Autodesk Inventor part; units mm, degrees
ref_plane "Work Plane1" through (0, 21, 0) normal (0, 1, 0) x (1, 0, 0)
ref_plane "YZ Plane" through (0, 0, 0) normal (1, 0, 0) x (0, 1, 0)
ref_plane "XZ Plane" through (0, 0, 0) normal (0, 1, 0) x (-1, 0, 0)
sketch "Sketch1" plane through (0, 0, 0) normal (0, 1, 0) x (-1, 0, 0)
  line L0 (8.2, 0) -> (8.2, -35)
  line L1 (8.2, -35) -> (-8.2, -35)
  line L2 (-8.2, -35) -> (-8.2, 0)
  line L3 (-8.2, 0) -> (0, 0)
  line L4 (0, 0) -> (8.2, 0)
  line L5 (-8.2, 0) -> (-14.5, 0)
  line L6 (-14.5, 0) -> (-14.5, -40)
  line L7 (-14.5, -40) -> (14.5, -40)
  line L8 (14.5, -40) -> (14.5, 0)
  line L9 (14.5, 0) -> (8.2, 0)
  line L10 (5.1, 0) -> (5.1, -30)
  line L11 (5.1, -30) -> (-5.1, -30)
  line L12 (-5.1, -30) -> (-5.1, 0)
  line L13 (-5.1, -30) -> (-8.2, -30) construction
  line L14 (5.1, -30) -> (8.2, -30) construction
  dimension "d2" = 5
  dimension "d17" = 5
  dimension "d26" = 29
  dimension "d27" = 10.2
  dimension "d28" = 16.4
  dimension "d29" = 40
extrude "Extrusion1" add sketch "Sketch1" along normal blind 42 contours L9 L8 L7 L6 L5 L2 L1 L0
sketch "Sketch2" plane through (14.5, 0, 0) normal (1, 0, 0) x (0, 0, -1)
  line L0 (0, 0) -> (40, 0)
  line L1 (40, 0) -> (40, 42)
  line L2 (0, 42) -> (40, 42)
  line L3 (0, 0) -> (0, 42)
  line L4 (0, 21) -> (0, 21) construction
  circle A0 centre (0, 21) radius 3.5
  line L5 (0, 21) -> (30, 21) construction
  circle A1 centre (30, 21) radius 3.5
  line L6 (0, 24.5) -> (30, 24.5)
  line L7 (30, 17.5) -> (0, 17.5)
  line L8 (0, 0) -> (0, 42)
  point P0 (0, 21)
  dimension "d6" = 7
  dimension "d8" = 0
  dimension "d40" = 30
extrude "Extrusion2" cut sketch "Sketch2" along normal blind 3.2 from surface at -6.3 contours A0 L3 | L3 A0 | A0 L6 A1 L7 | A1
sketch "Sketch3" plane through (14.5, 0, -40) normal (0, 0, -1) x (-1, 0, 0)
  line L0 (0, 0) -> (29, 0)
  line L1 (29, 0) -> (29, 42)
  line L2 (0, 42) -> (29, 42)
  line L3 (0, 0) -> (0, 42)
  line L4 (29, 0) -> (29, 42) construction
  line L5 (29, 21) -> (14.5, 21) construction
  line L6 (14.5, 21) -> (14.5, 0) construction
  circle A0 centre (14.5, 21) radius 1.9
  dimension "d11" = 3.8
extrude "Extrusion3" cut sketch "Sketch3" against normal blind 10 contours A0
extrude "Extrusion4" add sketch "Sketch1" along normal blind 11 contours L0 L1 L2 L3 L12 L11 L10 L4
extrude "Extrusion5" add sketch "Sketch1" along normal blind 3 contours L10 L11 L12 L3 L4
chamfer "Chamfer1" distance 2 angle 45 3 edges at (-5.1, 3, -15) (0, 3, -30) (5.1, 3, -15)
chamfer "Chamfer2" distance 2 angle 45 2 edges at (-6.65, 11, 0) (6.65, 11, 0)
ref_plane "Work Plane1" through (0, 21, 0) normal (0, 1, 0) x (1, 0, 0)
mirror "Mirror1" about plane through (0, 21, 0) normal (0, 1, 0) of "Extrusion4", "Extrusion5", "Chamfer1", "Chamfer2"
sketch "Sketch4" plane through (0, 42, 0) normal (0, 1, 0) x (1, 0, 0)
  line L0 (-14.5, 0) -> (14.5, 0)
  line L1 (14.5, 0) -> (14.5, 40)
  line L2 (14.5, 40) -> (-14.5, 40)
  line L3 (-14.5, 40) -> (-14.5, 0)
  line L4 (0, 0) -> (0, 10) construction
  circle A0 centre (0, 10) radius 1.5
  line L5 (0, 10) -> (0, 30) construction
  circle A1 centre (0, 30) radius 1.5
  dimension "d30" = 3
  dimension "d31" = 10
  dimension "d32" = 20
extrude "Extrusion6" cut sketch "Sketch4" against normal up to surface (3 mm away) contours A0 | A1
sketch "Sketch5" plane through (14.5, 0, -40) normal (0, 0, -1) x (-1, 0, 0)
  circle A0 centre (14.5, 21) radius 1.9
  line L0 (0, 0) -> (29, 0)
  line L1 (29, 0) -> (29, 42)
  line L2 (0, 42) -> (29, 42)
  line L3 (0, 0) -> (0, 42)
  line L4 (14.5, 0) -> (14.5, 8) construction
  line L5 (14.5, 8) -> (22, 8) construction
  line L6 (14.5, 8) -> (7, 8) construction
  circle A1 centre (7, 8) radius 1.5
  circle A2 centre (22, 8) radius 1.5
  dimension "d35" = 8
  dimension "d36" = 3
  dimension "d39" = 15
extrude "Extrusion7" cut sketch "Sketch5" against normal blind 6 contours A1 | A2
mirror "Mirror2" about plane through (0, 21, 0) normal (0, 1, 0) of "Extrusion6", "Extrusion7"
mirror "Mirror3" about plane through (0, 0, 0) normal (1, 0, 0) of "Extrusion2"
properties part number "tensionerholder_3DPrint"
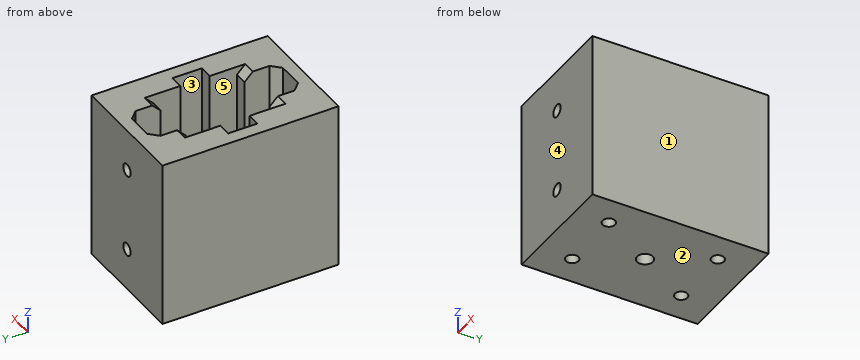
Input: part model. Units: mm. Frame: model coordinates. Face numbers are marked on the shaded views. A direction names the side the tool comes from. Round coordinates to 2 decimals unless told otherwise and drop trailing zeros. Write each loop counter-clockwise with the first axis right and the second up, starting at its lowest first coordinate (ties: lowest second). Pieces come first, ordered by that corner, then holes. Notation, with made-up numbers: M -3,71 L 16,71 A32 cw 16,97 Z; hole C -8.75,15 d2. An arc over 180 degrees is marked long. Write each question's results on one line, items separated by ' | '.
Q1. Section query B-B (y = 21). Return loops of the section in (x, z).
Results:
outline: M -14.5,-40 L -1.9,-40 L -1.9,-35 L -8.2,-35 L -8.2,-33.5 L -11.4,-33.5 L -11.4,0 L -14.5,0 Z; M 1.9,-40 L 14.5,-40 L 14.5,0 L 11.4,0 L 11.4,-33.5 L 8.2,-33.5 L 8.2,-35 L 1.9,-35 Z
Q2. Line query: line 1 along Y through (x, z) = (-7.5, -36.25); line 2 along X through (y, z) = (34, -38); line 3 along Y through (x, z) = (-11, -2). Output: solid intervals per line, ascending.
Results:
line 1: y = 0 to 6.5, 9.5 to 32.5, 35.5 to 42 | line 2: x = -14.5 to -9, -6 to 6, 9 to 14.5 | line 3: y = 0 to 17.5, 24.5 to 42
Q3. Access query for the marked faces 4 and 5. Directions: +Z, -Z, +X, -X, +Y, -Y. A direction counts if a zero-diameter tool reaches every point of the face in a straight line with its end or side. Return the directions, or none.
Results:
face 4: +Z, -Z, +X, -X, -Y | face 5: +Z
Q4. Pin query (flat end, axial travel): P1, Ø2.5, axis at x = 7.5, y = 34, coming from the -Z side. Return the tip coordinate at first contact, or that it passes through.
Results:
P1: stops at z = -34
Q5. Section query D-D (y = 8). Return loops of the section in (x, z), and give its area (3 significant figures).
Results:
outline: M -14.5,-40 L -9,-40 L -9,-34 L -6,-34 L -6,-40 L 6,-40 L 6,-34 L 9,-34 L 9,-40 L 14.5,-40 L 14.5,0 L 5.1,0 L 5.1,-30 L -5.1,-30 L -5.1,0 L -14.5,0 Z | area: 818 mm^2
Q6. Draft query along X for the marked faces 1, 2 and 3. Return one class per face: released by +X, released by -X, zero draft, split by the parting line, or undercut.
Results:
face 1: released by +X | face 2: zero draft | face 3: undercut
Q7. Section query C-C (x = 7.5). Return loops of the section in (y, z).
Results:
outline: M 0,-40 L 6.5,-40 L 6.5,-34 L 9.5,-34 L 9.5,-40 L 32.5,-40 L 32.5,-34 L 35.5,-34 L 35.5,-40 L 42,-40 L 42,0 L 33,0 L 31,-2 L 31,-35 L 11,-35 L 11,-2 L 9,0 L 0,0 Z
Q8. Section query A-A (z = -7). Return loops of the section in (x, y), and give its area (3 significant figures).
Results:
outline: M -14.5,0 L 14.5,0 L 14.5,42 L -14.5,42 Z; hole M -11.4,17.5 L -8.2,17.5 L -8.2,11 L -5.1,11 L -5.1,5 L -3.1,3 L 3.1,3 L 5.1,5 L 5.1,11 L 8.2,11 L 8.2,17.5 L 11.4,17.5 L 11.4,24.5 L 8.2,24.5 L 8.2,31 L 5.1,31 L 5.1,37 L 3.1,39 L -3.1,39 L -5.1,37 L -5.1,31 L -8.2,31 L -8.2,24.5 L -11.4,24.5 Z | area: 690 mm^2
